from build123d import *

# Parameters (mm, degrees)
SKETCH1_W                  = 168
SKETCH1_H                  = 120
BOSS_EXTRUDE1_DEPTH        = 20
SKETCH2_W                  = 168
SKETCH2_H                  = 104
CUT_EXTRUDE1_DEPTH         = 15
SKETCH3_R                  = 1.75
CUT_EXTRUDE2_DEPTH         = 21
SKETCH5_W                  = 2
SKETCH5_H                  = 40
BOSS_EXTRUDE2_DEPTH        = 8
SKETCH6_R                  = 1.75
CUT_EXTRUDE3_DEPTH         = 162.85
SKETCH7_W                  = 8
SKETCH7_H                  = 3
BOSS_EXTRUDE3_DEPTH        = 8
CHAMFER1_SIZE              = 5
LPATTERN1_COUNT            = 7
LPATTERN1_PITCH            = 24
CHAMFER1_OF_LPATTERN1_SIZE = 5


with BuildPart() as part:
    # Sketch1 → Boss-Extrude1 (new body)
    with BuildSketch(Plane.XY):
        Rectangle(SKETCH1_W, SKETCH1_H)
    extrude(amount=BOSS_EXTRUDE1_DEPTH)

    # Sketch2 → Cut-Extrude1 (cut)
    with BuildSketch(Plane.XY.offset(20)):
        with Locations((0, -8)):
            Rectangle(SKETCH2_W, SKETCH2_H)
    extrude(amount=-CUT_EXTRUDE1_DEPTH, mode=Mode.SUBTRACT)

    # Sketch3 → Cut-Extrude2 (cut, through all)
    with BuildSketch(Plane.XY.offset(20)):
        with Locations((-64, 52)):
            Circle(SKETCH3_R)
        with Locations((-34, 52)):
            Circle(SKETCH3_R)
        with Locations((-4, 52)):
            Circle(SKETCH3_R)
        with Locations((26, 52)):
            Circle(SKETCH3_R)
        with Locations((56, 52)):
            Circle(SKETCH3_R)
    extrude(amount=-CUT_EXTRUDE2_DEPTH, mode=Mode.SUBTRACT)

    # Sketch5 → Boss-Extrude2 (add)
    with BuildSketch(Plane.XY.offset(5)):
        with Locations((-76.85, -35)):
            Rectangle(SKETCH5_W, SKETCH5_H)
    boss_extrude2 = extrude(amount=BOSS_EXTRUDE2_DEPTH)

    # Sketch6 → Cut-Extrude3 (cut, through all)
    with BuildSketch(Plane.ZY.offset(77.85)):
        with Locations((10, -45)):
            Circle(SKETCH6_R)
        with Locations((10, -38.5)):
            Circle(SKETCH6_R)
        with Locations((10, -32)):
            Circle(SKETCH6_R)
    cut_extrude3 = extrude(amount=-CUT_EXTRUDE3_DEPTH, mode=Mode.SUBTRACT)

    # Sketch7 → Boss-Extrude3 (add)
    with BuildSketch(Plane.XY.offset(5)):
        with Locations((-74.85, -53.5)):
            Rectangle(SKETCH7_W, SKETCH7_H)
        with Locations((-74.85, -16.5)):
            Rectangle(SKETCH7_W, SKETCH7_H)
    boss_extrude3 = extrude(amount=BOSS_EXTRUDE3_DEPTH)

    # Chamfer1
    chamfer1_edges = [part.edges().sort_by_distance(p)[0] for p in [
        (-70.85, -16.5, 13),
        (-70.85, -53.5, 13),
    ]]
    chamfer(chamfer1_edges, length=CHAMFER1_SIZE)

    # LPattern1: Boss-Extrude2, Cut-Extrude3, Boss-Extrude3 ×7
    with Locations(*[(i * LPATTERN1_PITCH, 0, 0) for i in range(1, LPATTERN1_COUNT)]):
        add(boss_extrude2)
        add(cut_extrude3, mode=Mode.SUBTRACT)
        add(boss_extrude3)

    # Chamfer1 of LPattern1
    chamfer1_of_lpattern1_edges = [part.edges().sort_by_distance(p)[0] for p in [
        (-46.85, -16.5, 13),
        (-46.85, -53.5, 13),
        (-22.85, -16.5, 13),
        (-22.85, -53.5, 13),
        (1.15, -16.5, 13),
        (1.15, -53.5, 13),
        (25.15, -16.5, 13),
        (25.15, -53.5, 13),
        (49.15, -16.5, 13),
        (49.15, -53.5, 13),
        (73.15, -16.5, 13),
        (73.15, -53.5, 13),
    ]]
    chamfer(chamfer1_of_lpattern1_edges, length=CHAMFER1_OF_LPATTERN1_SIZE)


solid = part.part
Geometry check sheet. Reference: the model listing, model coordinates, mm. A direction names the side the tool comes from. Coordinates: 2 decimals unless noted, no trailing zeros. Order: outer loops, then holes, each group sorted by start corner. A loop starts at its lowest first (then second) coordinate and runs counter-clockwise, first axis right, second up. Notation, with made-up numbers: (69.5, 30) -> (109.5, 30) arc R10 cw to (109.5, 41) -> close; hole circle Ø5 at (-22.5, 21.5). An arc over 180 degrees is marked (long way). Use a Markdown table: item, result. Add a question column.
1. Go/stop test with flat-tipped pins: pin 1 Ø1.5 at (y, z) = (-53.5, 6.5) entering from +X; pin 2 Ø2.5 at (y, z) = (-29, 9) entering from -X; pin 3 Ø0.9 at (y, z) = (-16.5, 10) entering from -X. Record where each tip stops, or that it passes through.
2. Mould release check, pull along X, two halves, no side actions. Record for faces 1 (the face through (-74, -18, 8)), 2 (the face through (43.14, -40.21, 9.62)), 3 (the face through (46, -52, 8)), 4 (the face through (84, 13, 3)): pulls with the +X half, pulls with the -X half, needs draft (parallel to the pull), parting line crosses it, or undercut.
3. Cross-section at D-D (x = 35). Enter the section's corners in (y, z), and give its area (3 significant figures).
4. Cross-section at B-B (x = -34). Enter the section's corners in (y, z), and give its area (3 significant figures).
5. Cross-section at A-A (y = 52). Enter the section's corners in (x, z), and give its area (3 significant figures).
6. Set-up check for faces 5 (the face through (-4, -15, 8)), 6 (the face through (22, -52, 8)), 7 (the face through (-49.315, -16.521, 10.465)), 8 (the face through (-77.85, -35, 9)), 9 (the face through (70.685, -16.521, 10.465)): record each of +Z, -Z, +X, -X, +Y, -Y from which the full face is reachable in a straight line by a thin tool's end or side.
7. Material ranges on L1, parallel to Y at x = -52.85, z = 10; L2, parallel to Y at x = -1, z = 10; L3, parallel to Y at x = 62, z = 9, recorded low to high.
8. Cross-section at C-C (z = 15.5). Enter the section's corners in (x, y).
Filled sheet:
| question | item | result |
|---|---|---|
| 1 | pin 1 | x = 73.15 |
| 1 | pin 2 | x = -77.85 |
| 1 | pin 3 | x = -78.85 |
| 2 | face 1 | undercut |
| 2 | face 2 | needs draft |
| 2 | face 3 | undercut |
| 2 | face 4 | pulls with the +X half |
| 3 | outline | (-60, 0) -> (60, 0) -> (60, 20) -> (44, 20) -> (44, 5) -> (-60, 5) -> close |
| 3 | area | 840 mm2 |
| 4 | outline | (-60, 0) -> (50.25, 0) -> (50.25, 20) -> (44, 20) -> (44, 5) -> (-60, 5) -> close; (53.75, 0) -> (60, 0) -> (60, 20) -> (53.75, 20) -> close |
| 4 | area | 770 mm2 |
| 5 | outline | (-84, 0) -> (-65.75, 0) -> (-65.75, 20) -> (-84, 20) -> close; (-62.25, 0) -> (-35.75, 0) -> (-35.75, 20) -> (-62.25, 20) -> close; (-32.25, 0) -> (-5.75, 0) -> (-5.75, 20) -> (-32.25, 20) -> close; (-2.25, 0) -> (24.25, 0) -> (24.25, 20) -> (-2.25, 20) -> close; (27.75, 0) -> (54.25, 0) -> (54.25, 20) -> (27.75, 20) -> close; (57.75, 0) -> (84, 0) -> (84, 20) -> (57.75, 20) -> close |
| 5 | area | 3,010 mm2 |
| 6 | face 5 | +Z, +X, -X |
| 6 | face 6 | +Z |
| 6 | face 7 | +Z, -Y |
| 6 | face 8 | +Z, -X |
| 6 | face 9 | +Z, +X, -Y |
| 7 | L1 | -55 to -46.75, -43.25 to -40.25, -36.75 to -33.75, -30.25 to -15, 44 to 60 |
| 7 | L2 | -55 to -52, -18 to -15, 44 to 60 |
| 7 | L3 | 44 to 60 |
| 8 | outline | (-84, 44) -> (84, 44) -> (84, 60) -> (-84, 60) -> close; hole circle Ø3.5 at (-64, 52); hole circle Ø3.5 at (-34, 52); hole circle Ø3.5 at (-4, 52); hole circle Ø3.5 at (26, 52); hole circle Ø3.5 at (56, 52) |
